Check sheet for the modelled part. Datum: model origin and axes. Units: mm. A direction names the side the tool comes from. Coordinates: 2 decimals unless noted, no trailing zeros. Loops run counter-clockwise (first coordinate to the right, second up) from the corner with the lowest first, then second, coordinate; pieces in that order, holes last.
from build123d import *

# Parameters (mm, degrees)
SALIENTE_EXTRUIR1_DEPTH = 18
SALIENTE_EXTRUIR2_START = 1.5
CROQUIS2_R              = 2.7
SALIENTE_EXTRUIR2_DEPTH = 1.5
SALIENTE_EXTRUIR3_DEPTH = 1.5
CROQUIS6_W              = 5.4
CROQUIS6_H              = 1.803822617
SALIENTE_EXTRUIR7_DEPTH = 10
CROQUIS10_W             = 5.4
CROQUIS10_H             = 10
CORTAR_EXTRUIR3_DEPTH   = 10
CROQUIS12_W             = 50.345864286
CROQUIS12_H             = 43.398115734
CORTAR_EXTRUIR4_DEPTH   = 30
CROQUIS14_W             = 2
CROQUIS14_H             = 3
CORTAR_EXTRUIR5_DEPTH   = 30
CROQUIS15_W             = 3
CROQUIS15_H             = 9.965395542
CROQUIS15_H_2           = 4.625035451
CORTAR_EXTRUIR6_DEPTH   = 7.4
CROQUIS16_W             = 3.7
CROQUIS16_H             = 3
REVOLUCI_N2_ANGLE       = 180
CROQUIS17_W             = 0.5
CROQUIS17_H             = 9
REVOLUCI_N3_ANGLE       = 180


with BuildPart() as part:
    # Croquis1 → Saliente-Extruir1 (new body)
    with BuildSketch(Plane.XY):
        with BuildLine():
            Line((-53.667784589, 33.4650382), (-54.417784589, 34.764076306))
            Line((-54.417784589, 34.764076306), (-59.613937012, 31.764076306))
            ThreePointArc((-59.613937012, 31.764076306), (-73.945502317, 40.827707086), (-87.584573208, 30.752047693))
            Line((-87.584573208, 30.752047693), (-88.334573208, 29.453009587))
            Line((-88.334573208, 29.453009587), (-83.138420786, 26.453009587))
            ThreePointArc((-83.138420786, 26.453009587), (-83.82197264, 9.509694567), (-68.276660199, 2.735742387))
            Line((-68.276660199, 2.735742387), (-66.776660199, 2.735742387))
            Line((-66.776660199, 2.735742387), (-66.776660199, 8.735742387))
            ThreePointArc((-66.776660199, 8.735742387), (-51.761543041, 16.615426627), (-53.667784589, 33.4650382))
        make_face()
        with BuildLine():
            Line((-54.507549641, 31.745180452), (-55.016343575, 32.626437397))
            Line((-55.016343575, 32.626437397), (-60.212495998, 29.626437397))
            ThreePointArc((-60.212495998, 29.626437397), (-72.508207296, 39.071771198), (-85.675250182, 30.884718699))
            Line((-85.675250182, 30.884718699), (-86.184044116, 30.003461754))
            Line((-86.184044116, 30.003461754), (-80.987891693, 27.003461754))
            ThreePointArc((-80.987891693, 27.003461754), (-83.019935064, 11.632396511), (-69.346218174, 4.322929129))
            Line((-69.346218174, 4.322929129), (-68.328630306, 4.322929129))
            Line((-68.328630306, 4.322929129), (-68.328630306, 10.322929129))
            ThreePointArc((-68.328630306, 10.322929129), (-54.000875637, 16.248660571), (-54.507549641, 31.745180452))
        make_face(mode=Mode.SUBTRACT)
    extrude(amount=SALIENTE_EXTRUIR1_DEPTH)

    # Croquis2 → Saliente-Extruir2 (add)
    with BuildSketch(Plane(origin=(0, 0, 0), x_dir=(-1, 0, 0), z_dir=(0, 0, -1)).offset(SALIENTE_EXTRUIR2_START)):
        with BuildLine():
            Line((87.584573208, 30.752047693), (88.334573208, 29.453009587))
            Line((88.334573208, 29.453009587), (83.138420786, 26.453009587))
            ThreePointArc((83.138420786, 26.453009587), (83.82197264, 9.509694567), (68.276660199, 2.735742387))
            Line((68.276660199, 2.735742387), (66.776660199, 2.735742387))
            Line((66.776660199, 2.735742387), (66.776660199, 8.735742387))
            ThreePointArc((66.776660199, 8.735742387), (51.761543041, 16.615426627), (53.667784589, 33.4650382))
            Line((53.667784589, 33.4650382), (54.417784589, 34.764076306))
            Line((54.417784589, 34.764076306), (59.613937012, 31.764076306))
            ThreePointArc((59.613937012, 31.764076306), (73.945502317, 40.827707086), (87.584573208, 30.752047693))
        make_face()
        with Locations((69.843005999, 22.317609427)):
            Circle(CROQUIS2_R, mode=Mode.SUBTRACT)
    extrude(amount=-SALIENTE_EXTRUIR2_DEPTH)

    # Croquis3 → Saliente-Extruir3 (add)
    with BuildSketch(Plane.XY.offset(18)):
        with BuildLine():
            Line((-66.776660199, 8.735742387), (-66.776660199, 2.735742387))
            Line((-66.776660199, 2.735742387), (-68.276660199, 2.735742387))
            ThreePointArc((-68.276660199, 2.735742387), (-83.82197264, 9.509694567), (-83.138420786, 26.453009587))
            Line((-83.138420786, 26.453009587), (-88.334573208, 29.453009587))
            Line((-88.334573208, 29.453009587), (-87.584573208, 30.752047693))
            ThreePointArc((-87.584573208, 30.752047693), (-73.945502317, 40.827707086), (-59.613937012, 31.764076306))
            Line((-59.613937012, 31.764076306), (-54.417784589, 34.764076306))
            Line((-54.417784589, 34.764076306), (-53.667784589, 33.4650382))
            ThreePointArc((-53.667784589, 33.4650382), (-51.761543041, 16.615426627), (-66.776660199, 8.735742387))
        make_face()
    extrude(amount=SALIENTE_EXTRUIR3_DEPTH)

    # Croquis6 → Saliente-Extruir7 (add)
    with BuildSketch(Plane(origin=(0, 0, -1.5), x_dir=(-1, 0, 0), z_dir=(0, 0, -1))):
        with Locations((69.843005999, 21.415698119)):
            Rectangle(CROQUIS6_W, CROQUIS6_H)
    extrude(amount=SALIENTE_EXTRUIR7_DEPTH)

    # Croquis10 → Cortar-Extruir3 (cut)
    with BuildSketch(Plane(origin=(0, 22.317609427, 0), x_dir=(1, 0, 0), z_dir=(0, 1, 0))):
        with Locations((-69.843005999, 6.5)):
            Rectangle(CROQUIS10_W, CROQUIS10_H)
    extrude(amount=-CORTAR_EXTRUIR3_DEPTH, mode=Mode.SUBTRACT)

    # Croquis11 → Revolución1 (revolve)
    with BuildSketch(Plane(origin=(0, 22.317609427, 0), x_dir=(1, 0, 0), z_dir=(0, 1, 0)), mode=Mode.PRIVATE) as revoluci_n1_sk:
        Polygon((-72.543005999, 1.5), (-79.543005999, 1.5), (-72.543005999, 11.5), align=None)
        Polygon((-71.193005999, -19.5), (-69.843005999, -19.5), (-69.843005999, -26.5), (-71.193005999, -26.5), (-79.543005999, -26.5), (-79.543005999, -19.5), align=None)
    revolve(revoluci_n1_sk.sketch.rotate(Axis((-69.843005999, 22.317609427, 19.5), (0, 0, 1)), 180), axis=Axis((-69.843005999, 22.317609427, 19.5), (0, 0, 1)))

    # Croquis12 → Cortar-Extruir4 (cut)
    with BuildSketch(Plane(origin=(0, 22.317609427, 0), x_dir=(1, 0, 0), z_dir=(0, 1, 0))):
        with Locations((-66.462924906, -7.850212976)):
            Rectangle(CROQUIS12_W, CROQUIS12_H)
    extrude(amount=-CORTAR_EXTRUIR4_DEPTH, mode=Mode.SUBTRACT)

    # Croquis14 → Cortar-Extruir5 (cut)
    with BuildSketch(Plane.XZ.offset(-22.317609427)):
        with Locations((-74.543005999, -4)):
            Rectangle(CROQUIS14_W, CROQUIS14_H)
        with Locations((-65.143005999, -4)):
            Rectangle(CROQUIS14_W, CROQUIS14_H)
        with Locations((-65.143005999, 23)):
            Rectangle(CROQUIS14_W, CROQUIS14_H)
        with Locations((-74.543005999, 23)):
            Rectangle(CROQUIS14_W, CROQUIS14_H)
    extrude(amount=-CORTAR_EXTRUIR5_DEPTH, mode=Mode.SUBTRACT)

    # Croquis15 → Cortar-Extruir6 (cut)
    with BuildSketch(Plane(origin=(-66.143005999, 0, 0), x_dir=(0, 0, -1), z_dir=(1, 0, 0))):
        with Locations((4, 33.124395109)):
            Rectangle(CROQUIS15_W, CROQUIS15_H)
        with Locations((-23, 32.834394335)):
            Rectangle(CROQUIS15_W, CROQUIS15_H_2)
    extrude(amount=-CORTAR_EXTRUIR6_DEPTH, mode=Mode.SUBTRACT)

    # Croquis16 → Revolución2 (revolve)
    with BuildSketch(Plane.XZ.offset(-22.317609427)):
        with Locations((-71.693005999, 16.5)):
            Rectangle(CROQUIS16_W, CROQUIS16_H)
    revolve(axis=Axis((-69.843005999, 22.317609427, 15), (0, 0, -1)), revolution_arc=REVOLUCI_N2_ANGLE)

    # Croquis17 → Revolución3 (revolve)
    with BuildSketch(Plane.XZ.offset(-22.317609427)):
        with Locations((-72.293005999, -7)):
            Rectangle(CROQUIS17_W, CROQUIS17_H)
    revolve(axis=Axis((-69.843005999, 22.317609427, 0), (0, 0, -1)), revolution_arc=REVOLUCI_N3_ANGLE)


solid = part.part
(1) Section check D-D, the plane y = 37. Enter the section's corners in (x, z).
(2) Scan lines: line 1 along Z through (x, y) = (-75, 32.75); line 2 along Z through (x, y) = (-67, 28.75); line 3 along X through (y, z) = (25.75, 7). Record each from-to range of solid material in increasing order.
(3) Section check B-B, the plane z = 19. Enter the section's corners in (x, y), plus the area to 3 significant figures.
(4) Set-up check for faces 5 (the face through (-73.543, 26, 23)), 6 (the face through (-70, 29, -2.5)), 7 (the face through (-72.28, 39.06, 8.87)), 8 (the face through (-69.63, 32.015, 25.284)): record each of +Z, -Z, +X, -X, +Y, -Y from which the full face is reachable in a straight line by a thin tool's end or side.
(5) Draft check along X on faces 1 (the face through (-73.543, 25, -4)), 2 (the face through (-84.403, 24.441, 8.853)), 3 (the face through (-69, 22.318, 16)), 4 (the face through (-57.578, 31.147, 8.874)). Enter one of: pulls with the +X half, pulls with the -X half, needs draft (parallel to the pull), parting line crosses it, or undercut.
(6) Section check A-A, the plane x = -84.5. Enter the section's corners in (y, z).
(7) Section check C-C, the plane z = -3.5. Enter the section's corners in (x, y), plus the area to 3 significant figures.
(8) Gauge pin test, flat ends, axial feed: P1, Ø1.5, axis at x = -84, y = 27, coming from the -Z side; P2, Ø8, axis at y = 33, z = 17, coming from the -X side; P3, Ø1.5, axis at y = 25.5, z = -3.5, coming from the +X side; P4, Ø1.5, axis at y = 38.5, z = -2.5, coming from the -X side. Record the tip position at first contact, or that the pin passes through.
Determined:
1. outline: (-83.43, -1.5) - (-63.38, -1.5) - (-63.38, 19.5) - (-83.43, 19.5) - close; hole (-80.43, 0) - (-65.93, 0) - (-65.93, 18) - (-80.43, 18) - close
2. line 1: z = -1.5 to 0, 18 to 19.5
2. line 2: z = -2.5 to 0, 18 to 26.5
2. line 3: x = -83.63 to -82, -51.99 to -50.16
3. outline: (-88.33, 29.45) - (-83.14, 26.45) arc R15.01 ccw to (-85.31, 22.32) - (-50.07, 22.32) arc R15.01 ccw to (-53.67, 33.47) - (-54.42, 34.76) - (-59.61, 31.76) arc R15.01 ccw to (-87.58, 30.75) - close
3. area: 521 mm2
4. face 5: +Y, -Y
4. face 6: +Y
4. face 7: none
4. face 8: +Z, +Y
5. face 1: undercut
5. face 2: pulls with the -X half
5. face 3: needs draft
5. face 4: undercut
6. outline: (22.32, -1.5) - (24.25, -1.5) - (24.25, 19.5) - (22.32, 19.5) - close; (27.24, -1.5) - (35.94, -1.5) - (35.94, 19.5) - (27.24, 19.5) - close; hole (29.03, 0) - (33.04, 0) - (33.04, 18) - (29.03, 18) - close
7. outline: (-78.14, 22.32) - (-75.54, 22.32) - (-75.54, 28.35) arc R8.3 ccw to start; (-73.54, 22.32) - (-72.04, 22.32) arc R2.2 cw to (-67.64, 22.32) - (-66.14, 22.32) - (-66.14, 28.14) - (-73.54, 28.14) - close; (-64.14, 22.32) - (-61.54, 22.32) arc R8.3 ccw to (-64.14, 28.35) - close
7. area: 57.2 mm2
8. P1: stops at z = -1.5
8. P2: stops at x = -88.33
8. P3: stops at x = -61.55
8. P4: passes through
